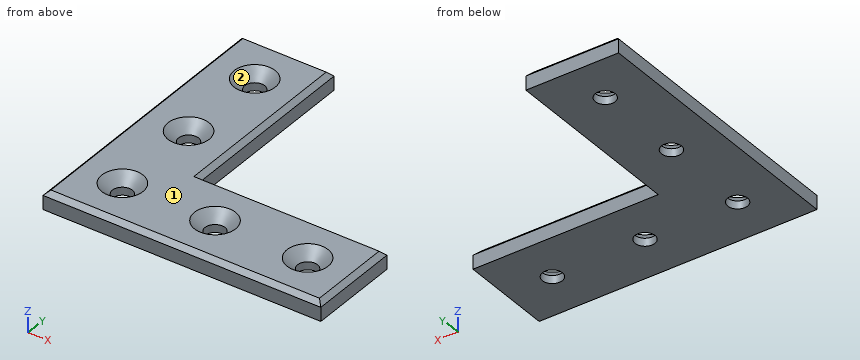
```python
from build123d import *

# Parameters (mm, degrees)
SKETCH1_R           = 2.15
BOSS_EXTRUDE1_DEPTH = 4
CHAMFER1_SIZE       = 1
CHAMFER2_SIZE       = 2.3


with BuildPart() as part:
    # Sketch1 → Boss-Extrude1 (new body)
    with BuildSketch(Plane.XY):
        Polygon((50, -10), (50, 10), (10, 10), (10, 50), (-10, 50), (-10, 10), (-10, -10), align=None)
        with Locations((0, 20)):
            Circle(SKETCH1_R, mode=Mode.SUBTRACT)
        with Locations((20, 0)):
            Circle(SKETCH1_R, mode=Mode.SUBTRACT)
        with Locations((0, 40)):
            Circle(SKETCH1_R, mode=Mode.SUBTRACT)
        Circle(SKETCH1_R, mode=Mode.SUBTRACT)
        with Locations((40, 0)):
            Circle(SKETCH1_R, mode=Mode.SUBTRACT)
    extrude(amount=BOSS_EXTRUDE1_DEPTH)

    # Chamfer1
    chamfer1_edges = [part.edges().sort_by_distance(p)[0] for p in [
        (0, 50, 4),
        (-10, 20, 4),
        (20, -10, 4),
        (50, 0, 4),
        (30, 10, 4),
        (10, 30, 4),
    ]]
    chamfer(chamfer1_edges, length=CHAMFER1_SIZE)

    # Chamfer2
    chamfer2_edges = [part.edges().sort_by_distance(p)[0] for p in [
        (17.85, 0, 4),
        (-2.15, 20, 4),
        (-2.15, 40, 4),
        (-2.15, 0, 4),
        (37.85, 0, 4),
    ]]
    chamfer(chamfer2_edges, length=CHAMFER2_SIZE)


solid = part.part
```
Geometry: final body of the model. Coordinates: model frame, mm. Face numbers are marked on the shaded views. Round coordinates to 2 decimals unless told otherwise and drop trailing zeros. Order: outer loops, then holes, each group sorted by start corner. A loop starts at its lowest first (then second) coordinate and runs counter-clockwise, first axis right, second up. Notation, with made-up numbers: (89, 64.25) -> (132, 64.25) arc R27 cw to (132, 90.25) -> close; hole circle Ø11 at (36.5, 76.5). An arc over 180 degrees is marked (long way). Use one line per item in the form item = value. Start each with the question number.
1. Pin query (flat end, axial travel): pin 1 Ø2 at (x, y) = (43, 1) entering from +Z; pin 2 Ø5.5 at (x, y) = (0, 20) entering from +Z; pin 3 Ø3.5 at (x, y) = (0, 0) entering from -Z; pin 4 Ø1.5 at (y, z) = (29.5, 2) entering from +X. Return the tip coordinate at first contact, or that it passes through.
2. Draft query along Y for the marked faces 1 and 2. Return one class per face: pulls with the +Y half, pulls with the -Y half, needs draft (parallel to the pull), parting line crosses it, or undercut.
3. Line query: probe 1 along Y at (x, z) = (0, 0.65); probe 2 along Y at (x, z) = (40, 0.95); probe 3 along X at (y, z) = (0.5, 1.85) (3 decimals). Output: solid intervals per line, ascending.
4. Cut plane A-A (z = 0.9). Return the cut outline in (x, y).
5. Cut plane B-B (x = 0). Return the cut outline in (y, z), then the cut area to 3 significant figures.
6. Cut plane C-C (y = 20). Return the cut outline in (x, z), then the cut area to 3 significant figures.
Solution:
q1.pin_1 = 3.71
q1.pin_2 = 2.3
q1.pin_3 = through
q1.pin_4 = 10
q2.face_1 = needs draft
q2.face_2 = undercut
q3.probe_1 = -10 to -2.15, 2.15 to 17.85, 22.15 to 37.85, 42.15 to 50
q3.probe_2 = -10 to -2.15, 2.15 to 10
q3.probe_3 = -10 to -2.245, 2.245 to 17.755, 22.245 to 37.755, 42.245 to 50
q4.outline = (-10, -10) -> (50, -10) -> (50, 10) -> (10, 10) -> (10, 50) -> (-10, 50) -> close; hole circle Ø4.3 at (0, 0); hole circle Ø4.3 at (0, 20); hole circle Ø4.3 at (0, 40); hole circle Ø4.3 at (20, 0); hole circle Ø4.3 at (40, 0)
q5.outline = (-10, 0) -> (-2.15, 0) -> (-2.15, 1.7) -> (-4.45, 4) -> (-9, 4) -> (-10, 3) -> close; (2.15, 0) -> (17.85, 0) -> (17.85, 1.7) -> (15.55, 4) -> (4.45, 4) -> (2.15, 1.7) -> close; (22.15, 0) -> (37.85, 0) -> (37.85, 1.7) -> (35.55, 4) -> (24.45, 4) -> (22.15, 1.7) -> close; (42.15, 0) -> (50, 0) -> (50, 3) -> (49, 4) -> (44.45, 4) -> (42.15, 1.7) -> close
q5.area = 172 mm^2
q6.outline = (-10, 0) -> (-2.15, 0) -> (-2.15, 1.7) -> (-4.45, 4) -> (-9, 4) -> (-10, 3) -> close; (2.15, 0) -> (10, 0) -> (10, 3) -> (9, 4) -> (4.45, 4) -> (2.15, 1.7) -> close
q6.area = 56.5 mm^2
